from build123d import *

# Parameters (mm, degrees)
F0_W     = 203.2
F0_H     = 203.2
F1_DEPTH = 12.7
F2_SIZE  = 1.524
F3_R     = 12.7
F4_DEPTH = 25.401
F5_R     = 12.7
F5_R_2   = 4.09575
F6_DEPTH = 12.7
F7_R     = 6.3754
F8_DEPTH = 6.35


# Not quite as in the source:
# - a pattern or mirror of a feature is missing from the dataset's text; its kind, count and spacing are read off the source's solid


with BuildPart() as f1:
    # F0 (on Front) → F1 (new body, symmetric)
    with BuildSketch(Plane.XZ):
        Rectangle(F0_W, F0_H)
    extrude(amount=F1_DEPTH, both=True)

    # F2
    f2_edges = [f1.edges().sort_by_distance(p)[0] for p in [
        (101.6, -12.7, 0),
        (0, -12.7, 101.6),
        (-101.6, -12.7, 0),
        (0, -12.7, -101.6),
    ]]
    chamfer(f2_edges, length=F2_SIZE)

    # F3 (on face) → F4 (cut, through all)
    with BuildSketch(Plane.XZ.offset(12.7)):
        with Locations((-50.8, -50.8)):
            Circle(F3_R)
    f4 = extrude(amount=-F4_DEPTH, mode=Mode.SUBTRACT)

    # F4_copies: F4 across plane
    add(f4.mirror(Plane.XY), mode=Mode.SUBTRACT)

    # F5 (on face) → F6 (join)
    with BuildSketch(Plane.XZ.offset(12.7)):
        with Locations((-50.8, 50.8)):
            Circle(F5_R)
        with Locations((-50.8, 50.8)):
            Circle(F5_R_2, mode=Mode.SUBTRACT)
        with Locations((-50.8, -50.8)):
            Circle(F5_R)
        with Locations((-50.8, -50.8)):
            Circle(F5_R_2, mode=Mode.SUBTRACT)
    extrude(amount=-F6_DEPTH)

    # F7 (on face) → F8 (cut)
    with BuildSketch(Plane.XZ.offset(12.7)):
        with Locations((-50.8, 50.8)):
            Circle(F7_R)
        with Locations((-50.8, -50.8)):
            Circle(F7_R)
    extrude(amount=-F8_DEPTH, mode=Mode.SUBTRACT)


solid = f1.part
Geometry check sheet. Reference: the model listing, model coordinates, mm. A direction names the side the tool comes from. Give positions to 0.01 mm unless a question says otherwise; leave off trailing zeros. Order: outer loops, then holes, each group sorted by start corner. A loop starts at its lowest first (then second) coordinate and runs counter-clockwise, first axis right, second up.
1) Cross-section at B-B (x = -50.8). Give the number of separate pieces and of enclosed holes in the cut face, then the cut area to 3 significant figures.
Results are:
separate pieces: 3
enclosed holes: 0
area: 4,250 mm2
2) Material ranges on probe 1 along Z at (x, y) = (-50.8, 3.25); probe 2 along Z at (x, y) = (-50.8, -3.5), recorded low to high.
Results are:
probe 1: z = -101.6 to -63.5, -38.1 to 38.1, 63.5 to 101.6
probe 2: z = -101.6 to -54.9, -46.7 to 46.7, 54.9 to 101.6
3) Gauge pin test, flat ends, axial feed: pin 1 (6.5 mm diameter, centred on x = -50.5, z = -49.5, fed in from -Y); pin 2 (20.5 mm diameter, centred on x = -50.8, z = 50.8, fed in from +Y). Record the tip position at first contact, or that the pin passes through.
Results are:
pin 1: stops at y = -6.35
pin 2: stops at y = 0
4) Cross-section at A-A (z = -50.8). Record the boundary of the cut face in (x, y), then the cut area to 3 significant figures.
Results are:
outline: (-101.6, -11.18) - (-100.08, -12.7) - (-57.18, -12.7) - (-57.18, -6.35) - (-54.9, -6.35) - (-54.9, 0) - (-63.5, 0) - (-63.5, 12.7) - (-101.6, 12.7) - close; (-46.7, -6.35) - (-44.42, -6.35) - (-44.42, -12.7) - (100.08, -12.7) - (101.6, -11.18) - (101.6, 12.7) - (-38.1, 12.7) - (-38.1, 0) - (-46.7, 0) - close
area: 4,700 mm2
5) Cross-section at C-C (y = 4). Record the boundary of the cut face in (x, z), then the cut area to 3 significant figures.
Results are:
outline: (-101.6, -101.6) - (101.6, -101.6) - (101.6, 101.6) - (-101.6, 101.6) - close; hole circle Ø25.4 at (-50.8, -50.8); hole circle Ø25.4 at (-50.8, 50.8)
area: 40,300 mm2
6) Tool access check on faces 1 (the flat face through (-46.6, -6.35, 49.5)), 2 (the flat face through (-1, 1, 101.6)), 3 (the cylindrical face through (-44.94, 6.261, 62.067)). Record the directions out of +Z, -Z, +X, -X, +Y, -Y that give a thin tool (end or side, any length) a straight path to the whole face; none if there is none.
Results are:
face 1: -Y
face 2: +Z, +X, -X, +Y, -Y
face 3: +Y
7) Draft check along X on faces 4 (the flat face through (101.6, 1, -1)), 5 (the flat face through (-46.6, -6.35, -52.1)), 6 (the flat face through (-1, 12.7, 1)). Enter one of: released by +X, released by -X, zero draft, split by the parting line, or undercut.
Results are:
face 4: released by +X
face 5: undercut
face 6: zero draft
